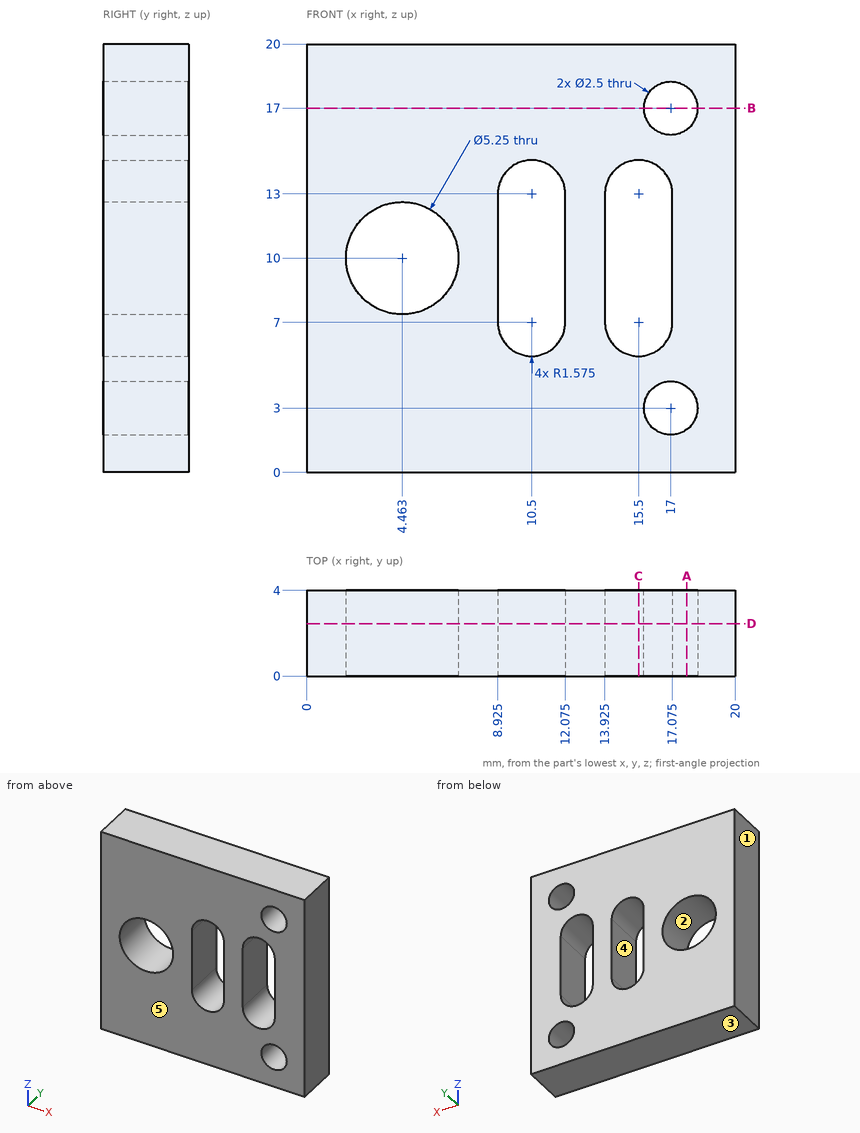
Source: three-view drawing plus pictorial views. Frame: mm from the lowest corner of the part. A direction names the side the tool comes from. Coordinates: 2 decimals unless noted, no trailing zeros. Write each loop counter-clockwise with the first axis right and the second up, starting at its lowest first coordinate (ties: lowest second). Pieces come first, ordered by that corner, then holes. Notation, with made-up numbers: (32, 4) -> (74, 4) arc R27 ccw to (74, 24) -> close; hole circle Ø10 at (49.25, 66). An arc over 180 degrees is marked (long way). Answer as a JSON object with one key per item and string values.
1. Section C-C on x = 15.5. Return the cut outline in (y, z) (1 decimal), then the cut area to 3 significant figures.
Result set:
{"outline": "(0, 0) -> (4, 0) -> (4, 5.4) -> (0, 5.4) -> close; (0, 14.6) -> (4, 14.6) -> (4, 20) -> (0, 20) -> close", "area": "43.4 mm2"}
2. Material intervals for line 1 (X direction, y = 2.15, z = 17); line 2 (X direction, y = 2.35, z = 6.75) (1 decimal); line 3 (Z direction, x = 6.25, y = 1.4) (1 decimal), sorted ascending. Write a range as from..to.
Result set:
{"line 1": "x = 0..15.75, 18.25..20", "line 2": "x = 0..8.9, 12.1..13.9, 17.1..20", "line 3": "z = 0..8.1, 11.9..20"}
3. Section B-B on z = 17. Return the cut outline in (x, y).
Result set:
{"outline": "(0, 0) -> (15.75, 0) -> (15.75, 4) -> (0, 4) -> close; (18.25, 0) -> (20, 0) -> (20, 4) -> (18.25, 4) -> close"}
4. Section A-A on x = 17.75. Return the cut outline in (y, z).
Result set:
{"outline": "(0, 0) -> (4, 0) -> (4, 2) -> (0, 2) -> close; (0, 4) -> (4, 4) -> (4, 16) -> (0, 16) -> close; (0, 18) -> (4, 18) -> (4, 20) -> (0, 20) -> close"}
5. First-contact query: P1, Ø4, axis at x = 16, z = 6, coming from the -Y side; P2, Ø2, axis at x = 17, z = 17, coming from the +Y side. Flat tips, straight axial feed; report the tip coordinate or a pass-through.
Result set:
{"P1": "stops at y = 0", "P2": "passes through"}
6. Section D-D on y = 2.45. Count the separate pieces of the cut face and the enclosed holes in it, then the cut area to 3 significant figures.
Result set:
{"separate pieces": "1", "enclosed holes": "5", "area": "315 mm2"}
7. Access query for the marked faces 4 and 5. Directions: +Z, -Z, +X, -X, +Y, -Y. A direction counts if a zero-diameter tool reaches every point of the face in a straight line with its end or side. Return the directions, or none.
Result set:
{"face 4": "+Y, -Y", "face 5": "+Z, -Z, +X, -X, -Y"}
8. Mould query, pull axis Z, two halves, no side actions, for the marked faces 1, 2 and 3. Classes: released by +Z, released by -Z, zero draft, split by the parting line, or undercut.
Result set:
{"face 1": "zero draft", "face 2": "undercut", "face 3": "released by -Z"}
